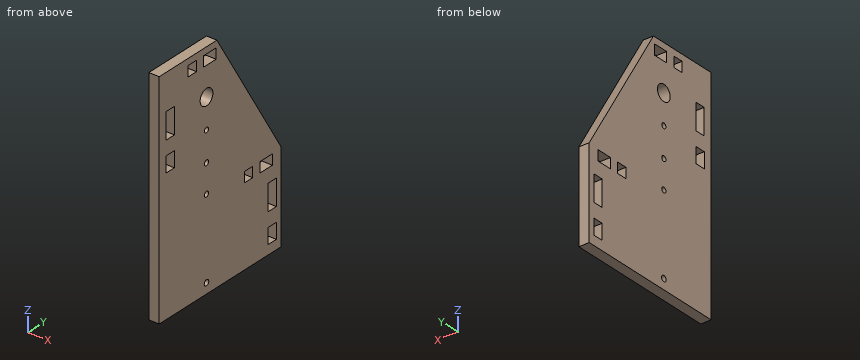
```python
from build123d import *

# Parameters (mm, degrees)
SKETCH1_R           = 3.075
SKETCH1_R_2         = 1
SKETCH1_R_3         = 1.1
SKETCH1_W           = 10
SKETCH1_H           = 4
SKETCH1_W_2         = 4
SKETCH1_H_2         = 6
SKETCH1_W_3         = 6
BOSS_EXTRUDE1_DEPTH = 4


with BuildPart() as part:
    # Sketch1 → Boss-Extrude1 (new body)
    with BuildSketch(Plane(origin=(0, 0, 0), x_dir=(0, 0, -1), z_dir=(1, 0, 0))):
        Polygon((-45.126561274, -21.465862465), (41.462435166, -21.465862465), (41.462435166, 37.538855), (6.497816801, 37.538855), (-45.126561274, 6.437068625), align=None)
        with Locations((-27.502183199, 1.424311927)):
            Circle(SKETCH1_R, mode=Mode.SUBTRACT)
        with Locations((-16.002183199, 1.424311927)):
            Circle(SKETCH1_R_2, mode=Mode.SUBTRACT)
        with Locations((-4.502183199, 1.424311927)):
            Circle(SKETCH1_R_2, mode=Mode.SUBTRACT)
        with Locations((6.497816801, 1.424311927)):
            Circle(SKETCH1_R_2, mode=Mode.SUBTRACT)
        with Locations((37.497816801, 1.424311927)):
            Circle(SKETCH1_R_3, mode=Mode.SUBTRACT)
        with Locations((21.33035671, 33.233983224)):
            Rectangle(SKETCH1_W, SKETCH1_H, mode=Mode.SUBTRACT)
        with Locations((-40.626561274, 3.062484248)):
            Rectangle(SKETCH1_W_2, SKETCH1_H_2, mode=Mode.SUBTRACT)
        with Locations((-40.626561274, -5.437515752)):
            Rectangle(SKETCH1_W_2, SKETCH1_H, mode=Mode.SUBTRACT)
        with Locations((-26.374737007, -16.111091518)):
            Rectangle(SKETCH1_W, SKETCH1_H, mode=Mode.SUBTRACT)
        with Locations((-12.874826786, -16.142516965)):
            Rectangle(SKETCH1_W_3, SKETCH1_H, mode=Mode.SUBTRACT)
        with Locations((34.83035671, 33.233983224)):
            Rectangle(SKETCH1_W_3, SKETCH1_H, mode=Mode.SUBTRACT)
        with Locations((8.963743124, 30.24228943)):
            Rectangle(SKETCH1_W_2, SKETCH1_H_2, mode=Mode.SUBTRACT)
        with Locations((8.963743124, 21.74228943)):
            Rectangle(SKETCH1_W_2, SKETCH1_H, mode=Mode.SUBTRACT)
    extrude(amount=BOSS_EXTRUDE1_DEPTH)


solid = part.part
```
Input: part model. Units: mm. Frame: model coordinates. Give positions to 0.01 mm unless a question says otherwise; leave off trailing zeros. Order: outer loops, then holes, each group sorted by start corner. A loop starts at its lowest first (then second) coordinate and runs counter-clockwise, first axis right, second up. Notation, with made-up numbers: M 22,-14 L 41,-14 A21 ccw 41,-1 Z; hole C 87,-23 d10. An arc over 180 degrees is marked long. One line per question, with ' | ' between items. Start each with the question number.
1. Section query A-A (y = 22.5). Return the cut outline in (x, z), and give its area (3 significant figures).
2. Section query B-B (z = 14). Return the cut outline in (x, y), and give its area (3 significant figures).
3. Section query D-D (y = 12). Return the cut outline in (x, z), and give its area (3 significant figures).
4. Section query C-C (x = 1.9). Count the separate pieces of the cut face and the enclosed holes in it, and give its area (3 significant figures).
5. Material intervals for probe 1 along Y at (x, z) = (1.4, -9.5); probe 2 along Z at (x, y) = (2.85, 5); probe 3 along Y at (x, z) = (0.85, -22), sorted ascending. Write a range as [from, to].
Here are the results:
1) outline: M 0,-41.46 L 4,-41.46 L 4,-10.96 L 0,-10.96 Z; M 0,-6.96 L 4,-6.96 L 4,18.46 L 0,18.46 Z | area: 224 mm²
2) outline: M 0,-21.47 L 4,-21.47 L 4,-18.14 L 0,-18.14 Z; M 0,-14.14 L 4,-14.14 L 4,25.19 L 0,25.19 Z | area: 171 mm²
3) outline: M 0,-41.46 L 4,-41.46 L 4,35.89 L 0,35.89 Z | area: 309 mm²
4) separate pieces: 1 | enclosed holes: 13 | area: 4,060 mm²
5) probe 1: [-21.47, 19.74], [23.74, 27.24], [33.24, 37.54] | probe 2: [-41.46, 38.63], [42.63, 45.13] | probe 3: [-21.47, 31.23], [35.23, 37.54]
